The model under review builds one solid part; all positions refer to its coordinate system, in mm. Face numbers are marked on the shaded views. A direction names the side the tool comes from. Round coordinates to 2 decimals unless told otherwise and drop trailing zeros. Loops run counter-clockwise (first coordinate to the right, second up) from the corner with the lowest first, then second, coordinate; pieces in that order, holes last. Notation, with made-up numbers: (-21.75, -4) -> (28.25, -4) arc R30 ccw to (28.25, 22) -> close; hole circle Ø3 at (-26.5, 75.25). An arc over 180 degrees is marked (long way). Use a Markdown table: item, result. Add a question column.
1) For the marked faces 1, 2 and 3, list the 3-axis set-ups (+Z, -Z, +X, -X, +Y, -Y) from which the entire face can be reached by the end or side of a thin tool; tool diameter is ignored.
2) Consider section B-B on x = 45. Give the boundary of the cut face in (y, z), plus the area to 3 significant figures.
3) Consider section C-C on y = 21.5. Give the boundary of the cut face in (x, z), plus the area to 4 significant figures.
4) Insertion check: pin 1 (1.5 mm diameter, centred on x = 25.5, y = 40.5, fed in from +Z); pin 2 (6 mm diameter, centred on x = 41, z = 9, fed in from +Y); pin 3 (6 mm diameter, centred on x = 9.5, z = 20.5, fed in from +Y). Each pin has a flat end and moves straight along its axis. Give the tip position at first contact, or say it passes through.
5) Consider section A-A on z = 11. Give the boundary of the cut face in (x, y).
6) Wall thickness on probe 1 along Y at (x, z) = (8.5, 44); probe 2 along Y at (x, z) = (54, 7): over which ranges is each line inside the solid? List them lowest first.
7) Consider section D-D on x = 65.5. Give the boundary of the cut face in (y, z), plus the area to 4 significant figures.
from build123d import *

# Parameters (mm, degrees)
SKETCH1_W           = 80
SKETCH1_H           = 50
BOSS_EXTRUDE1_DEPTH = 50
CUT_EXTRUDE1_DEPTH  = 50
CUT_EXTRUDE2_DEPTH  = 30


with BuildPart() as part:
    # Sketch1 → Boss-Extrude1 (new body)
    with BuildSketch(Plane.XY):
        with Locations((40, 25)):
            Rectangle(SKETCH1_W, SKETCH1_H)
    extrude(amount=BOSS_EXTRUDE1_DEPTH)

    # Sketch2 → Cut-Extrude1 (cut)
    with BuildSketch(Plane.XY.offset(50)):
        Polygon((70, 50), (60, 40), (20, 40), (0, 20), (0, 50), align=None)
    extrude(amount=-CUT_EXTRUDE1_DEPTH, mode=Mode.SUBTRACT)

    # Sketch3 → Cut-Extrude2 (cut)
    with BuildSketch(Plane.XY.offset(50)):
        Polygon((0, 20), (40, 20), (60, 40), (20, 40), align=None)
    extrude(amount=-CUT_EXTRUDE2_DEPTH, mode=Mode.SUBTRACT)


solid = part.part
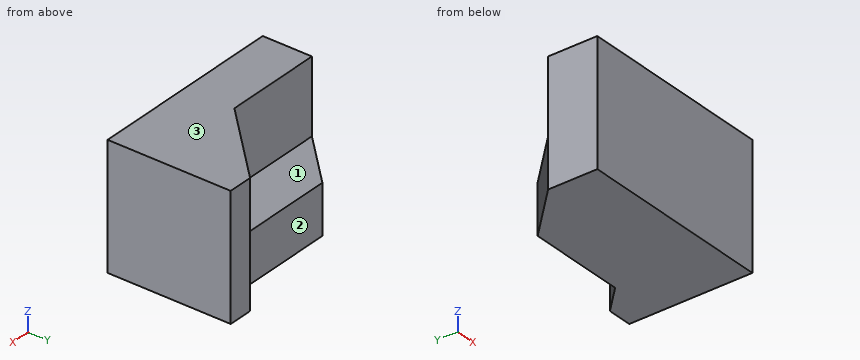
Result set:
| question | item | result |
|---|---|---|
| 1 | face 1 | +Z, -X, +Y |
| 1 | face 2 | +Z, -Z, -X, +Y |
| 1 | face 3 | +Z, +X, -X, +Y, -Y |
| 2 | outline | (0, 0) -> (40, 0) -> (40, 20) -> (25, 20) -> (25, 50) -> (0, 50) -> close |
| 2 | area | 1,550 mm2 |
| 3 | outline | (1.5, 0) -> (80, 0) -> (80, 50) -> (41.5, 50) -> (41.5, 20) -> (1.5, 20) -> close |
| 3 | area | 2,725 mm2 |
| 4 | pin 1 | z = 20 |
| 4 | pin 2 | y = 40 |
| 4 | pin 3 | y = 32.46 |
| 5 | outline | (0, 0) -> (80, 0) -> (80, 50) -> (70, 50) -> (60, 40) -> (20, 40) -> (0, 20) -> close |
| 6 | probe 1 | 0 to 20 |
| 6 | probe 2 | 0 to 40 |
| 7 | outline | (0, 0) -> (45.5, 0) -> (45.5, 50) -> (0, 50) -> close |
| 7 | area | 2,275 mm2 |
